Work out the finished part from the listing and answer in its coordinate system (mm). A direction names the side the tool comes from. Coordinates: 2 decimals unless noted, no trailing zeros. Loops run counter-clockwise (first coordinate to the right, second up) from the corner with the lowest first, then second, coordinate; pieces in that order, holes last. Notation, with made-up numbers: (81.5, 37.25) -> (98.5, 37.25) arc R12 ccw to (98.5, 42.25) -> close; hole circle Ø5 at (-34.5, 70.5). An arc over 180 degrees is marked (long way). Use a Markdown table: item, result. Add a question column.
```python
from build123d import *

# Parameters (mm, degrees)
F1_DEPTH  = 3.175
F2_R      = 1.016
F3_W      = 24.9555
F3_H      = 0.4668365944
F3_W_2    = 8.3583763037
F3_W_3    = 6.5895795759
F4_DEPTH  = 1.5875
F5_R      = 1.524
F6_DEPTH  = 25.4
F5_R_2    = 3.175
F7_DEPTH  = 1.5875
F9_W      = 1.294683665
F9_H      = 1.482822001
F10_DEPTH = 2.8222222222
F11_R     = 0.79375
F12_DEPTH = 5.08
F13_R     = 0.254
F15_DEPTH = 2.8222222222


# Not quite as in the source:
# - a fillet or chamfer that OpenCascade refuses, or shapes differently, is made with other operations: its cross-section is extruded or revolved along the edge and cut away or added


with BuildPart() as f1:
    # F0 (on Top) → F1 (new body)
    with BuildSketch(Plane.XY):
        with BuildLine():
            ThreePointArc((0, 1.5875), (0.4649679849, 0.4649679849), (1.5875, 0))
            Line((1.5875, 0), (25.4, 0))
            ThreePointArc((25.4, 0), (26.5225320151, 0.4649679849), (26.9875, 1.5875))
            Line((26.9875, 1.5875), (26.9875, 26.9875))
            ThreePointArc((26.9875, 26.9875), (24.7424359697, 27.9174359697), (23.8125, 30.1625))
            Line((23.8125, 30.1625), (23.8125, 32.7025))
            ThreePointArc((23.8125, 32.7025), (22.8825640303, 34.9475640303), (20.6375, 35.8775))
            Line((20.6375, 35.8775), (6.35, 35.8775))
            ThreePointArc((6.35, 35.8775), (4.1049359697, 34.9475640303), (3.175, 32.7025))
            Line((3.175, 32.7025), (3.175, 30.1625))
            ThreePointArc((3.175, 30.1625), (2.2450640303, 27.9174359697), (0, 26.9875))
            Line((0, 26.9875), (0, 1.5875))
        make_face()
    extrude(amount=F1_DEPTH)

    # F2
    f2_edges = [f1.edges().sort_by_distance(p)[0] for p in [
        (26.9875, 14.2875, 3.175),
        (3.175, 31.4325, 3.175),
        (2.245064, 27.917436, 3.175),
        (24.742436, 27.917436, 3.175),
        (23.8125, 31.4325, 3.175),
        (22.882564, 34.947564, 3.175),
        (13.49375, 35.8775, 3.175),
        (4.104936, 34.947564, 3.175),
    ]]
    fillet(f2_edges, radius=F2_R)

    # F3 (on face) → F4 (cut)
    with BuildSketch(Plane.XY.offset(3.175)):
        with BuildLine():
            Line((43.3063970949, 12.1285), (25.9715, 12.1285))
            Line((25.9715, 12.1285), (25.9715, 1.5875))
            ThreePointArc((25.9715, 1.5875), (25.8041115254, 1.1833884746), (25.4, 1.016))
            Line((25.4, 1.016), (14.0335, 1.016))
            Line((14.0335, 1.016), (14.0335, -10.401187452))
            Line((14.0335, -10.401187452), (43.3063970949, -10.401187452))
            Line((43.3063970949, -10.401187452), (43.3063970949, 12.1285))
        make_face()
        with BuildLine():
            Line((25.9715, 12.1285), (14.0335, 12.1285))
            Line((14.0335, 12.1285), (14.0335, 1.016))
            Line((14.0335, 1.016), (25.4, 1.016))
            ThreePointArc((25.4, 1.016), (25.8041115254, 1.1833884746), (25.9715, 1.5875))
            Line((25.9715, 1.5875), (25.9715, 12.1285))
        make_face()
        with BuildLine():
            Line((1.5875, 1.016), (12.954, 1.016))
            Line((12.954, 1.016), (12.954, 12.1285))
            Line((12.954, 12.1285), (1.016, 12.1285))
            Line((1.016, 12.1285), (1.016, 1.5875))
            ThreePointArc((1.016, 1.5875), (1.1833884746, 1.1833884746), (1.5875, 1.016))
        make_face()
        with BuildLine():
            Line((12.954, -10.9148975462), (12.954, 1.016))
            Line((12.954, 1.016), (1.5875, 1.016))
            ThreePointArc((1.5875, 1.016), (1.1833884746, 1.1833884746), (1.016, 1.5875))
            Line((1.016, 1.5875), (1.016, 12.1285))
            Line((1.016, 12.1285), (-5.5735795759, 12.1285))
            Line((-5.5735795759, 12.1285), (-5.5735795759, -10.9148975462))
            Line((-5.5735795759, -10.9148975462), (12.954, -10.9148975462))
        make_face()
        with Locations((13.49375, 13.6085897574)):
            Rectangle(F3_W, F3_H)
        with Locations((30.1506881518, 13.6085897574)):
            Rectangle(F3_W_2, F3_H)
        with Locations((-2.2787897879, 13.6085897574)):
            Rectangle(F3_W_3, F3_H)
    extrude(amount=-F4_DEPTH, mode=Mode.SUBTRACT)

    # F5 (on face) → F6 (cut)
    with BuildSketch(Plane.XY.offset(3.175)):
        with Locations((13.49375, 20.5581425011)):
            Circle(F5_R)
    extrude(amount=-F6_DEPTH, mode=Mode.SUBTRACT)

    # F5 (on face) → F7 (join)
    with BuildSketch(Plane.XY.offset(3.175)):
        with Locations((13.49375, 20.5581425011)):
            Circle(F5_R_2)
        with Locations((13.49375, 20.5581425011)):
            Circle(F5_R, mode=Mode.SUBTRACT)
    extrude(amount=F7_DEPTH)

    # F8: fillet of radius 2.54 on 1 edges, made by hand

    # F8_s1 → F8_t2 (revolve, cut)
    with BuildSketch(Plane.XZ.offset(-20.5581425011)):
        with BuildLine():
            ThreePointArc((15.01775, 2.3831557626), (15.4709270559, 3.8311785525), (16.66875, 4.7625))
            Line((16.66875, 4.7625), (15.01775, 4.7625))
            Line((15.01775, 4.7625), (15.01775, 2.3831557626))
        make_face()
    revolve(axis=Axis((13.49375, 20.5581425011, 4.7625), (0, 0, 1)), mode=Mode.SUBTRACT)

    # F9 (on face) → F10 (cut)
    with BuildSketch(Plane(origin=(0, 0, 0), x_dir=(1, 0, 0), z_dir=(0, 0, -1))):
        with BuildLine():
            ThreePointArc((15.1753826067, -15.5802866697), (17.8362583784, -17.462592513), (18.8565061088, -20.5581425011))
            Line((18.8565061088, -20.5581425011), (26.1830221862, -20.5581425011))
            Line((26.1830221862, -20.5581425011), (26.1830221862, -15.5802866697))
            Line((26.1830221862, -15.5802866697), (15.1753826067, -15.5802866697))
        make_face()
        with BuildLine():
            Line((26.1830221862, -20.5581425011), (18.8565061088, -20.5581425011))
            ThreePointArc((18.8565061088, -20.5581425011), (17.8362583784, -23.6536924892), (15.1753826067, -25.5359983325))
            Line((15.1753826067, -25.5359983325), (24.8883385211, -25.5359983325))
            Line((24.8883385211, -25.5359983325), (24.8883385211, -24.0531763315))
            Line((24.8883385211, -24.0531763315), (26.1830221862, -24.0531763315))
            Line((26.1830221862, -24.0531763315), (26.1830221862, -20.5581425011))
        make_face()
        with Locations((25.5356803536, -24.794587332)):
            Rectangle(F9_W, F9_H)
        with BuildLine():
            Line((12.1251240555, -15.5802866697), (1.117484476, -15.5802866697))
            Line((1.117484476, -15.5802866697), (1.117484476, -20.5581425011))
            Line((1.117484476, -20.5581425011), (1.117484476, -25.5359983325))
            Line((1.117484476, -25.5359983325), (12.1251240555, -25.5359983325))
            ThreePointArc((12.1251240555, -25.5359983325), (8.4440005534, -20.5581425011), (12.1251240555, -15.5802866697))
        make_face()
    extrude(amount=-F10_DEPTH, mode=Mode.SUBTRACT)

    # F11 (on face) → F12 (join)
    with BuildSketch(Plane(origin=(0, 0, 2.8222222222), x_dir=(1, 0, 0), z_dir=(0, 0, -1))):
        with Locations((22.4790647626, -20.5581425011)):
            Circle(F11_R)
        with Locations((4.8214418996, -21.3518925011)):
            Circle(F11_R)
    extrude(amount=F12_DEPTH)

    # F13
    f13_edges = [f1.edges().sort_by_distance(p)[0] for p in [
        (21.685315, 20.558143, -2.257778),
        (4.027692, 21.351893, -2.257778),
    ]]
    fillet(f13_edges, radius=F13_R)

    # F14 (on face) → F15 (cut)
    with BuildSketch(Plane(origin=(0, 0, 0), x_dir=(1, 0, 0), z_dir=(0, 0, -1))):
        with BuildLine():
            Line((10.4354891836, -27.7508334085), (3.8518141955, -27.7508334085))
            Line((3.8518141955, -27.7508334085), (3.8518141955, -29.2588919401))
            ThreePointArc((3.8518141955, -29.2588919401), (7.5132373167, -33.3483248509), (12.7214891836, -35.0814126432))
            Line((12.7214891836, -35.0814126432), (12.7214891836, -30.0368334085))
            ThreePointArc((12.7214891836, -30.0368334085), (12.0519352854, -28.4203873067), (10.4354891836, -27.7508334085))
        make_face()
        with BuildLine():
            ThreePointArc((14.0368680542, -35.0814126432), (19.2451199211, -33.3483248509), (22.9065430423, -29.2588919401))
            Line((22.9065430423, -29.2588919401), (22.9065430423, -27.7508334085))
            Line((22.9065430423, -27.7508334085), (16.3228680542, -27.7508334085))
            ThreePointArc((16.3228680542, -27.7508334085), (14.7064219524, -28.4203873067), (14.0368680542, -30.0368334085))
            Line((14.0368680542, -30.0368334085), (14.0368680542, -35.0814126432))
        make_face()
    extrude(amount=-F15_DEPTH, mode=Mode.SUBTRACT)


solid = f1.part
```
Item 1: Find the intervals of material crossed by probe 1 along Y at (x, z) = (14.5, 1.25); probe 2 along Y at (x, z) = (25, 2.5); probe 3 along X at (y, z) = (17.5, 0.25), in increasing order.
Item 2: For a pull along Y with two mould halves and no side action, classify faces 5 (the face through (0, 14, 1)), 6 (the face through (26.51, 0.45, 0.78)), 7 (the face through (22.907, 29, 1)) as +Y half, -Y half, draft (parallel to the pull), parting line (faces both ways), or undercut.
Item 3: For faces 1 (the face through (23.812, 31, 1)), 2 (the face through (21, 12.128, 2)), 3 (the face through (6, 6, 1.588)), 4 (the face through (9, 31, 2.822)), determine the directions among +Z, -Z, +X, -X, +Y, -Y from which every point of the face is accessible in a straight line to the end or side of a thin tool.
Item 4: Section C-C (z = 3.75) is taken. Determine the outline of the cut face in (x, y) (3 decimals).
Item 5: Section B-B (y = 9) is taken. Determine the outline of the cut face in (x, z) (1 decimal), then the cut area to 3 significant figures.
Item 6: Section D-D (y = 16) is taken. Determine the outline of the cut face in (x, z) (1 decimal), then the cut area to 3 significant figures.
Item 7: Given pin 1 (6 mm diameter, centred on x = 22, y = 4.5, fed in from +Z); pin 2 (2.5 mm diameter, centred on y = 31.5, z = 2, fed in from +X); pin 3 (2 mm diameter, centred on x = 9.5, y = 30, fed in from -Z), each flat-ended and moving along its own axis, determine where each tip first touches the part or whether it passes through.
Item 8: Section A-A (z = 0.5) is taken. Count the separate pieces of the cut face and the enclosed holes in it, then the cut area to 3 significant figures.
Output:
| question | item | result |
|---|---|---|
| 1 | probe 1 | y = 0 to 19.41, 21.7 to 28.66, 35.04 to 35.88 |
| 1 | probe 2 | y = 12.13 to 13.38, 13.84 to 15.58, 25.54 to 27.61 |
| 1 | probe 3 | x = 0 to 1.12, 9.44 to 17.86, 26.18 to 26.99 |
| 2 | face 5 | draft |
| 2 | face 6 | -Y half |
| 2 | face 7 | undercut |
| 3 | face 1 | +Z, -Z, +X, +Y |
| 3 | face 2 | +Z, +X, -Y |
| 3 | face 3 | +Z, -X, -Y |
| 3 | face 4 | -Z |
| 4 | outline | circle Ø6.35 at (13.494, 20.558); hole circle Ø3.846 at (13.494, 20.558) |
| 5 | outline | (0, 0) -> (27, 0) -> (27, 1.6) -> (14, 1.6) -> (14, 3.2) -> (13, 3.2) -> (13, 1.6) -> (0, 1.6) -> close |
| 5 | area | 44.6 mm2 |
| 6 | outline | (0, 0) -> (1.1, 0) -> (1.1, 2.8) -> (11.1, 2.8) -> (11.1, 0) -> (16.2, 0) -> (16.2, 2.8) -> (26.2, 2.8) -> (26.2, 0) -> (27, 0) -> (27, 2.2) arc R1 ccw to (26, 3.2) -> (1, 3.2) arc R1 ccw to (0, 2.2) -> close |
| 6 | area | 28.7 mm2 |
| 7 | pin 1 | stops at z = 1.59 |
| 7 | pin 2 | stops at x = 23.81 |
| 7 | pin 3 | stops at z = 2.82 |
| 8 | separate pieces | 3 |
| 8 | enclosed holes | 5 |
| 8 | area | 646 mm2 |
